```python
from build123d import *

# Parameters (mm, degrees)
SKETCH_2_R          = 2
SKETCH_2_R_2        = 1.5
SKETCH_2_W          = 20
SKETCH_2_H          = 2
EXTRUDE_1_DEPTH     = 3
SKETCH_3_R          = 0.75
CUT_EXTRUDE_1_DEPTH = 141.027398671
FILLET_1_R          = 5


with BuildPart() as part:
    # 草图2 → 凸台-拉伸1 (new body)
    with BuildSketch(Plane.XY):
        with BuildLine():
            Line((-132.601963201, -4.701034703), (-8.26765697, 12.828618462))
            ThreePointArc((-8.26765697, 12.828618462), (-4.434509027, 17.565346586), (-8.891400832, 21.720551987))
            Line((-8.891400832, 21.720551987), (-131.973846298, 21.720551987))
            Line((-131.973846298, 21.720551987), (-138.082164404, 1.709761493))
            ThreePointArc((-138.082164404, 1.709761493), (-137.100605417, -2.998907272), (-132.601963201, -4.701034703))
        make_face()
        with Locations((-59.03447946, 10.720551987)):
            Circle(SKETCH_2_R, mode=Mode.SUBTRACT)
        with Locations((-133.3, 0.25)):
            Circle(SKETCH_2_R, mode=Mode.SUBTRACT)
        with Locations((-125, 13.720551987)):
            Circle(SKETCH_2_R_2, mode=Mode.SUBTRACT)
        with Locations((-30, 13.720551987)):
            Circle(SKETCH_2_R_2, mode=Mode.SUBTRACT)
        with Locations((-70, 17.720551987)):
            Rectangle(SKETCH_2_W, SKETCH_2_H, mode=Mode.SUBTRACT)
        with Locations((-105, 17.720551987)):
            Rectangle(SKETCH_2_W, SKETCH_2_H, mode=Mode.SUBTRACT)
        with Locations((-35, 17.720551987)):
            Rectangle(SKETCH_2_W, SKETCH_2_H, mode=Mode.SUBTRACT)
    extrude(amount=EXTRUDE_1_DEPTH)

    # 草图3 → 切除-拉伸1 (cut, through all)
    with BuildSketch(Plane.XY.offset(3)):
        with Locations((-114.25, 18.720551987)):
            Circle(SKETCH_3_R)
        with Locations((-114.25, 16.720551987)):
            Circle(SKETCH_3_R)
        with Locations((-95.75, 18.720551987)):
            Circle(SKETCH_3_R)
        with Locations((-95.75, 16.720551987)):
            Circle(SKETCH_3_R)
        with Locations((-79.25, 18.720551987)):
            Circle(SKETCH_3_R)
        with Locations((-79.25, 16.720551987)):
            Circle(SKETCH_3_R)
        with Locations((-60.75, 18.720551987)):
            Circle(SKETCH_3_R)
        with Locations((-60.75, 16.720551987)):
            Circle(SKETCH_3_R)
        with Locations((-44.25, 18.720551987)):
            Circle(SKETCH_3_R)
        with Locations((-44.25, 16.720551987)):
            Circle(SKETCH_3_R)
        with Locations((-25.75, 18.720551987)):
            Circle(SKETCH_3_R)
        with Locations((-25.75, 16.720551987)):
            Circle(SKETCH_3_R)
        with BuildLine():
            Line((-116.854825567, 9.596408883), (-118.409147877, 4.504464164))
            ThreePointArc((-118.409147877, 4.504464164), (-118.114680182, 3.091863534), (-116.765087517, 2.581225305))
            Line((-116.765087517, 2.581225305), (-73.115887133, 8.735241576))
            ThreePointArc((-73.115887133, 8.735241576), (-71.828975077, 10.325514799), (-73.325298173, 11.720551987))
            Line((-73.325298173, 11.720551987), (-113.985526924, 11.720551987))
            ThreePointArc((-113.985526924, 11.720551987), (-115.770524027, 11.13173123), (-116.854825567, 9.596408883))
        make_face()
    extrude(amount=-CUT_EXTRUDE_1_DEPTH, mode=Mode.SUBTRACT)

    # 圆角1
    fillet_1_edges = [part.edges().sort_by_distance(p)[0] for p in [
        (-131.973846298, 21.720551987, 1.5),
    ]]
    fillet(fillet_1_edges, radius=FILLET_1_R)


solid = part.part
```
Design review of the part built by this model. Coordinates are the model's own, in mm. A direction names the side the tool comes from. Give positions to 0.01 mm unless a question says otherwise; leave off trailing zeros. Loops run counter-clockwise (first coordinate to the right, second up) from the corner with the lowest first, then second, coordinate; pieces in that order, holes last. Notation, with made-up numbers: M -27.5,52 L 22.5,52 A18 ccw 22.5,62 Z; hole C -38.75,-28.75 d4. An arc over 180 degrees is marked long. Return JSON: item names as keys, results as strings. Group by question number.
Item 1: We need section D-D (z = 2.1). Give the number of separate pieces and of enclosed holes in the cut face, and give its area (3 significant figures).
Item 2: We need section C-C (x = -30). Give the boundary of the cut face in (y, z).
Item 3: For probe 1 along X at (y, z) = (14.5, 1.4); probe 2 along X at (y, z) = (17, 1.35); probe 3 along Y at (x, z) = (-30, 1.25), list the stretches that pass through material, from the lowest coordinate up.
Item 4: We need section B-B (x = -125). Give the boundary of the cut face in (y, z).
Item 5: We need section A-A (x = -101). Give the boundary of the cut face in (y, z), and give its area (3 significant figures).
Item 6: Insertion check: pin 1 Ø1 at (y, z) = (18, 1) entering from +X; pin 2 Ø1 at (y, z) = (17.5, 1) entering from -X; pin 3 Ø0.6 at (y, z) = (17, 1.5) entering from -X. Each pin has a flat end and moves straight along its axis. Give the tip position at first contact, or say it passes through.
Item 7: Tool access review of faces 1 (the flat face through (-117.62, 7.09, 1.52)), 2 (the cylindrical face through (-4.43, 17.47, 1.48)): name each direction out of +Z, -Z, +X, -X, +Y, -Y from which nothing blocks a thin tool from reaching the whole face with its end or side.
Item 8: Mouldability with a two-part tool opening along X and no side actions: class faces 3 (the cylindrical face through (-31.11, 14.73, 1.48)), 4 (the flat face through (-68, 21.721, 1)), 5 (the cylindrical face through (-131.3, 20.7, 1.5)) as released by +X, released by -X, zero draft, split by the parting line, or undercut.
Output:
{
 "1": {"separate pieces": "1", "enclosed holes": "8", "area": "1,860 mm^2"},
 "2": {"outline": "M 9.76,0 L 12.22,0 L 12.22,3 L 9.76,3 Z; M 15.22,0 L 16.72,0 L 16.72,3 L 15.22,3 Z; M 18.72,0 L 21.72,0 L 21.72,3 L 18.72,3 Z"},
 "3": {"probe 1": "x = -134.18 to -126.28, -123.72 to -31.28, -28.72 to -5.37", "probe 2": "x = -133.41 to -115, -95 to -80, -60 to -45, -25 to -4.43", "probe 3": "y = 9.76 to 12.22, 15.22 to 16.72, 18.72 to 21.72"},
 "4": {"outline": "M -3.63,0 L 12.22,0 L 12.22,3 L -3.63,3 Z; M 15.22,0 L 21.72,0 L 21.72,3 L 15.22,3 Z"},
 "5": {"outline": "M -0.25,0 L 4.8,0 L 4.8,3 L -0.25,3 Z; M 11.72,0 L 16.72,0 L 16.72,3 L 11.72,3 Z; M 18.72,0 L 21.72,0 L 21.72,3 L 18.72,3 Z", "area": "39.1 mm^2"},
 "6": {"pin 1": "stops at x = -4.43", "pin 2": "stops at x = -133.41", "pin 3": "stops at x = -133.51"},
 "7": {"face 1": "+Z, -Z", "face 2": "+Z, -Z, +X"},
 "8": {"face 3": "undercut", "face 4": "zero draft", "face 5": "released by -X"}
}
